Work out the finished part from the listing and answer in its coordinate system (mm). Face numbers are marked on the shaded views. A direction names the side the tool comes from. Coordinates: 2 decimals unless noted, no trailing zeros. Write each loop counter-clockwise with the first axis right and the second up, starting at its lowest first coordinate (ties: lowest second). Pieces come first, ordered by that corner, then holes. Notation, with made-up numbers: (39.5, -2) - (78.5, -2) arc R22 cw to (78.5, 6) - close; hole circle Ø10 at (84.25, 34). An arc over 180 degrees is marked (long way). Use a Markdown table: item, result. Add a question column.
(1) A tool of negligible diameter and unlimited length cuts with its end or side. For the marked faces 1, 2 and 3, from which of +Z, -Z, +X, -X, +Y, -Y can it reach the whole face along a straight path? Write none if from no direction.
(2) The part is cut by section D-D, the plane z = 8.25. Give the vertices of the cut face in (x, y).
(3) The part is cut by section C-C, the plane y = -9.75. Give the vertices of the cut face in (x, z).
(4) Given pin 1 Ø6 at (x, y) = (-2.5, -17) entering from +Z; pin 2 Ø4 at (y, z) = (-19.5, 9.5) entering from +X; pin 3 Ø3 at (y, z) = (-19, 12.5) entering from -X; pin 4 Ø1.8 at (x, z) = (12.5, 10.5) entering from -Y, each flat-ended and moving along its own axis, determine where each tip first touches the part or whether it passes through.
(5) The part is cut by section B-B, the plane z = 13.75. Give the vertices of the cut face in (x, y), then the cut area to 3 significant figures.
(6) Find the intervals of material crossed by line 1 (Y direction, x = 7, z = 12); line 2 (Y direction, x = 11.75, z = 10); line 3 (X direction, y = -10, z = 12.25), in increasing order. Write a range as from..to.
(7) For a pull along Y with two mould halves and no side action, classify the marked faces 4, 5 and 6 as released by +Y, released by -Y, zero draft, split by the parting line, or undercut.
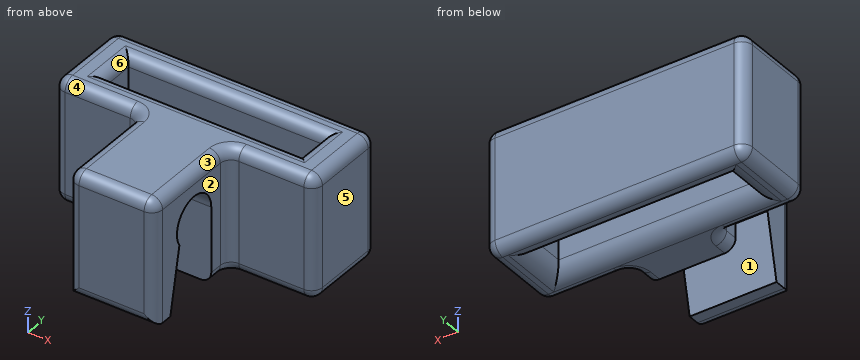
from build123d import *

# Parameters (mm, degrees)
F1_DEPTH = 8
F2_W     = 24
F2_H     = 11.337432079
F3_DEPTH = 8
F4_W     = 18
F4_H     = 3
F5_DEPTH = 11.338432079
F6_F1_R  = 1
F6_F2_R  = 1
F7_R     = 1.49999


# Not quite as in the source:
# - a fillet or chamfer is up to 0.001 mm smaller than in the source, because OpenCascade refuses the exact size


with BuildPart() as f1:
    # F0 (on Right) → F1 (new body)
    with BuildSketch(Plane.YZ):
        with BuildLine():
            ThreePointArc((-20.601621214, 10.7601184938), (-19.2613938683, 14.0777191086), (-16.4163531623, 11.9078281993))
            Line((-16.4163531623, 11.9078281993), (-16.4163531623, 4.9222996458))
            Line((-16.4163531623, 4.9222996458), (-14.2332110554, 4.9222996458))
            Line((-14.2332110554, 4.9222996458), (-14.2332110554, 16.2597317249))
            Line((-14.2332110554, 16.2597317249), (-23.8023772836, 16.2597317249))
            Line((-23.8023772836, 16.2597317249), (-23.8023772836, 4.9222996458))
            Line((-23.8023772836, 4.9222996458), (-21.7834785581, 4.9222996458))
            Line((-21.7834785581, 4.9222996458), (-20.601621214, 10.7601184938))
        make_face()
    extrude(amount=F1_DEPTH)

    # F2 (on face) → F3 (join)
    with BuildSketch(Plane(origin=(0, -14.2332110554, 0), x_dir=(-1, 0, 0), z_dir=(0, 1, 0))):
        with Locations((-4, 10.5910156853)):
            Rectangle(F2_W, F2_H)
    extrude(amount=F3_DEPTH)

    # F4 (on face) → F5 (cut, through all)
    with BuildSketch(Plane.XY.offset(16.2597317249)):
        with Locations((4, -10.2332110554)):
            Rectangle(F4_W, F4_H)
    extrude(amount=-F5_DEPTH, mode=Mode.SUBTRACT)

    # F6: fillet of radius 1 on 26 edges, made by hand

    # F6_f1
    f6_f1_edges = [f1.edges().sort_by_distance(p)[0] for p in [
        (0, -14.2332110554, 10.5910156853),
        (8, -14.2332110554, 10.5910156853),
    ]]
    fillet(f6_f1_edges, radius=F6_F1_R)

    # F6_f2
    f6_f2_edges = [f1.edges().sort_by_distance(p)[0] for p in [
        (-8, -10.2332110554, 16.2597317249),
        (-4.5, -14.2332110554, 16.2597317249),
        (4, -6.2332110554, 16.2597317249),
        (0, -19.5177941695, 16.2597317249),
        (16, -10.2332110554, 16.2597317249),
        (4, -23.8023772836, 16.2597317249),
        (12.5, -14.2332110554, 16.2597317249),
        (8, -19.5177941695, 16.2597317249),
        (-5, -10.2332110554, 16.2597317249),
        (4, -8.7332110554, 16.2597317249),
        (13, -10.2332110554, 16.2597317249),
        (4, -11.7332110554, 16.2597317249),
        (16, -10.2332110554, 4.9222996458),
        (16, -14.2332110554, 10.5910156853),
        (16, -6.2332110554, 10.5910156853),
        (4, -6.2332110554, 4.9222996458),
        (-8, -6.2332110554, 10.5910156853),
        (-8, -10.2332110554, 4.9222996458),
        (-8, -14.2332110554, 10.5910156853),
        (-4.5, -14.2332110554, 4.9222996458),
        (12.5, -14.2332110554, 4.9222996458),
        (4, -23.8023772836, 4.9222996458),
        (0, -23.8023772836, 10.5910156853),
        (8, -23.8023772836, 10.5910156853),
        (8.2928932188, -14.5261042742, 4.9222996458),
        (-0.2928932188, -14.5261042742, 4.9222996458),
        (8.2928932188, -14.5261042742, 16.2597317249),
        (-0.2928932188, -14.5261042742, 16.2597317249),
    ]]
    fillet(f6_f2_edges, radius=F6_F2_R)

    # F7 (radius 1.5 in the source; OpenCascade refuses exactly that, so slightly less here)
    f7_edges = [f1.edges().sort_by_distance(p)[0] for p in [
        (-5, -10.233211, 4.9223),
        (4, -11.733211, 4.9223),
        (4, -8.733211, 4.9223),
        (13, -10.233211, 4.9223),
    ]]
    fillet(f7_edges, radius=F7_R)


solid = f1.part
Model answer:
| question | item | result |
|---|---|---|
| 1 | face 1 | -Z, +X, -X |
| 1 | face 2 | +Z, -Z, +X, -Y |
| 1 | face 3 | +Z, +X, -Y |
| 2 | outline | (-8, -13.23) arc R1 ccw to (-7, -14.23) - (-1, -14.23) arc R1 cw to (0, -15.23) - (0, -16.42) - (8, -16.42) - (8, -15.23) arc R1 cw to (9, -14.23) - (15, -14.23) arc R1 ccw to (16, -13.23) - (16, -7.23) arc R1 ccw to (15, -6.23) - (-7, -6.23) arc R1 ccw to (-8, -7.23) - close; (0, -22.8) arc R1 ccw to (1, -23.8) - (7, -23.8) arc R1 ccw to (8, -22.8) - (8, -21.11) - (0, -21.11) - close; hole (-5, -11.73) - (13, -11.73) - (13, -8.73) - (-5, -8.73) - close |
| 3 | outline | (-8, 5.92) arc R1 ccw to (-7, 4.92) - (-6.5, 4.92) arc R1.5 ccw to (-5, 6.42) - (-5, 15.26) arc R1 ccw to (-6, 16.26) - (-7, 16.26) arc R1 ccw to (-8, 15.26) - close; (13, 6.42) arc R1.5 ccw to (14.5, 4.92) - (15, 4.92) arc R1 ccw to (16, 5.92) - (16, 15.26) arc R1 ccw to (15, 16.26) - (14, 16.26) arc R1 ccw to (13, 15.26) - close |
| 4 | pin 1 | z = 16.13 |
| 4 | pin 2 | x = 8 |
| 4 | pin 3 | through |
| 4 | pin 4 | y = -14.23 |
| 5 | outline | (-8, -13.23) arc R1 ccw to (-7, -14.23) - (-1, -14.23) arc R1 cw to (0, -15.23) - (0, -17.37) - (8, -17.37) - (8, -15.23) arc R1 cw to (9, -14.23) - (15, -14.23) arc R1 ccw to (16, -13.23) - (16, -7.23) arc R1 ccw to (15, -6.23) - (-7, -6.23) arc R1 ccw to (-8, -7.23) - close; (0, -22.8) arc R1 ccw to (1, -23.8) - (7, -23.8) arc R1 ccw to (8, -22.8) - (8, -19.96) - (0, -19.96) - close; hole (-5, -11.73) - (13, -11.73) - (13, -8.73) - (-5, -8.73) - close |
| 5 | area | 193 mm^2 |
| 6 | line 1 | -23.8..-20.91, -16.42..-11.73, -8.73..-6.23 |
| 6 | line 2 | -14.23..-11.73, -8.73..-6.23 |
| 6 | line 3 | -8..-5, 13..16 |
| 7 | face 4 | released by -Y |
| 7 | face 5 | zero draft |
| 7 | face 6 | undercut |
